Model file for the job. Use its own axes, mm. A direction names the side the tool comes from. Give positions to 0.01 mm unless a question says otherwise; leave off trailing zeros. Write each loop counter-clockwise with the first axis right and the second up, starting at its lowest first coordinate (ties: lowest second). Pieces come first, ordered by that corner, then holes. Notation, with made-up numbers: (72.25, -10) - (128.25, -10) arc R32 ccw to (128.25, 23) - close; hole circle Ø4 at (3, 42.5). An arc over 180 degrees is marked (long way). One line per item, written item: value. Start each with the question number.
(1) Mould opens along X. For faces 6 (the face through (-47.622, 0.74, 30.417)), 7 (the face through (65.665, 5.979, 35.509)), 8 (the face through (5, 2, 39.516)) say: pulls with the +X half, pulls with the -X half, needs draft (parallel to the pull), parting line crosses it, or undercut.
(2) Cut at A-A, the plane y = 6.25. List the corners of the cut face in (x, z), and give its area (3 significant figures).
(3) Cut at D-D, the plane z = 5. List the corners of the cut face in (x, y), and give its area (3 significant figures).
(4) Cut at C-C, the plane z = -14. List the corners of the cut face in (x, y), and give its area (3 significant figures).
(5) Drop flat-ended pins along their axis: P1, Ø5, axis at x = 60, z = -54.5, coming from the +Y side; P2, Ø1.8, axis at x = -49, z = -56, coming from the -Y side; P3, Ø0.9, axis at x = -16.5, y = 6.5, coming from the +Z side; P4, Ø1.8, axis at x = 59.52, z = 29.52, coming from the -Y side. Give the stop position or say it passes through.
(6) Cut at B-B, the plane x = 39.5. List the corners of the cut face in (y, z), and give its area (3 significant figures).
(7) Probe L1, parallel to X at y = 6.25, z = -35; L2, parallel to Z at x = 6, y = 6; L3, parallel to X at y = 0.5, z = 32. List the from-to ranges inside material, lowest first.
(8) 3-axis set-ups, long thin cutter, end or side, ignore diameter. For faces 1 (the face through (-56.63, 5.98, -61.48)), 2 (the face through (4, 6, -64.484)), 3 (the face through (34, 2, -21.699)), 4 (the face through (62.378, 0.74, 30.417)), 5 (the face through (64.665, 5.979, 34.509)): which of +Z, -Z, +X, -X, +Y, -Y reach the whole face in a straight line?
from build123d import *

# Parameters (mm, degrees)
SKETCH_1_R          = 6.5
EXTRUDE_1_DEPTH     = 4.5
EXTRUDE_2_DEPTH     = 3
SKETCH_3_R          = 1
CUT_EXTRUDE_1_DEPTH = 10
SKETCH_4_R          = 3
CUT_EXTRUDE_2_DEPTH = 1
SKETCH_5_R          = 3
CUT_EXTRUDE_3_DEPTH = 1.5
SKETCH_6_W          = 19.238645782
SKETCH_6_H          = 11.749776954
CUT_EXTRUDE_6_DEPTH = 10


with BuildPart() as part:
    # 草图1 → 凸台-拉伸1 (new body)
    with BuildSketch(Plane(origin=(0, 0, 0), x_dir=(1, 0, 0), z_dir=(0, 1, 0))):
        with BuildLine():
            Line((-50.483870968, 65.483870968), (59.516129032, 65.483870968))
            ThreePointArc((59.516129032, 65.483870968), (66.587196844, 62.55493878), (69.516129032, 55.483870968))
            Line((69.516129032, 55.483870968), (69.516129032, -29.516129032))
            ThreePointArc((69.516129032, -29.516129032), (66.587196844, -36.587196844), (59.516129032, -39.516129032))
            Line((59.516129032, -39.516129032), (-50.483870968, -39.516129032))
            ThreePointArc((-50.483870968, -39.516129032), (-57.55493878, -36.587196844), (-60.483870968, -29.516129032))
            Line((-60.483870968, -29.516129032), (-60.483870968, 55.483870968))
            ThreePointArc((-60.483870968, 55.483870968), (-57.55493878, 62.55493878), (-50.483870968, 65.483870968))
        make_face()
        with Locations((-0.483870968, 15.483870968)):
            Circle(SKETCH_1_R, mode=Mode.SUBTRACT)
    extrude(amount=EXTRUDE_1_DEPTH)

    # 草图2 → 凸台-拉伸2 (add)
    with BuildSketch(Plane(origin=(0, 4.5, 0), x_dir=(1, 0, 0), z_dir=(0, 1, 0))):
        with BuildLine():
            Line((-49.483870968, 64.483870968), (58.516129032, 64.483870968))
            ThreePointArc((58.516129032, 64.483870968), (65.587196844, 61.55493878), (68.516129032, 54.483870968))
            Line((68.516129032, 54.483870968), (68.516129032, -28.516129032))
            ThreePointArc((68.516129032, -28.516129032), (65.587196844, -35.587196844), (58.516129032, -38.516129032))
            Line((58.516129032, -38.516129032), (-49.483870968, -38.516129032))
            ThreePointArc((-49.483870968, -38.516129032), (-56.55493878, -35.587196844), (-59.483870968, -28.516129032))
            Line((-59.483870968, -28.516129032), (-59.483870968, 54.483870968))
            ThreePointArc((-59.483870968, 54.483870968), (-56.55493878, 61.55493878), (-49.483870968, 64.483870968))
        make_face()
        with BuildLine():
            Line((-48.483870968, 63.483870968), (57.516129032, 63.483870968))
            ThreePointArc((57.516129032, 63.483870968), (64.587196844, 60.55493878), (67.516129032, 53.483870968))
            Line((67.516129032, 53.483870968), (67.516129032, -27.516129032))
            ThreePointArc((67.516129032, -27.516129032), (64.587196844, -34.587196844), (57.516129032, -37.516129032))
            Line((57.516129032, -37.516129032), (-48.483870968, -37.516129032))
            ThreePointArc((-48.483870968, -37.516129032), (-55.55493878, -34.587196844), (-58.483870968, -27.516129032))
            Line((-58.483870968, -27.516129032), (-58.483870968, 53.483870968))
            ThreePointArc((-58.483870968, 53.483870968), (-55.55493878, 60.55493878), (-48.483870968, 63.483870968))
        make_face(mode=Mode.SUBTRACT)
    extrude(amount=EXTRUDE_2_DEPTH)

    # 草图3 → 切除-拉伸1 (cut)
    with BuildSketch(Plane(origin=(0, 4.5, 0), x_dir=(1, 0, 0), z_dir=(0, 1, 0))):
        with Locations((-50.483870968, 55.483870968)):
            Circle(SKETCH_3_R)
        with Locations((-50.483870968, -29.516129032)):
            Circle(SKETCH_3_R)
        with Locations((59.516129032, -29.516129032)):
            Circle(SKETCH_3_R)
        with Locations((59.516129032, 55.483870968)):
            Circle(SKETCH_3_R)
    extrude(amount=-CUT_EXTRUDE_1_DEPTH, mode=Mode.SUBTRACT)

    # 草图4 → 切除-拉伸2 (cut)
    with BuildSketch(Plane(origin=(0, 4.5, 0), x_dir=(1, 0, 0), z_dir=(0, 1, 0))):
        with Locations((-50.483870968, 55.483870968)):
            Circle(SKETCH_4_R)
        with Locations((59.516129032, 55.483870968)):
            Circle(SKETCH_4_R)
        with Locations((59.516129032, -29.516129032)):
            Circle(SKETCH_4_R)
        with Locations((-50.483870968, -29.516129032)):
            Circle(SKETCH_4_R)
    extrude(amount=-CUT_EXTRUDE_2_DEPTH, mode=Mode.SUBTRACT)

    # 草图5 → 切除-拉伸3 (cut)
    with BuildSketch(Plane.XZ):
        with Locations((-50.483870968, 29.516129032)):
            Circle(SKETCH_5_R)
        with Locations((59.516129032, 29.516129032)):
            Circle(SKETCH_5_R)
        with Locations((59.516129032, -55.483870968)):
            Circle(SKETCH_5_R)
        with Locations((-50.483870968, -55.483870968)):
            Circle(SKETCH_5_R)
    extrude(amount=-CUT_EXTRUDE_3_DEPTH, mode=Mode.SUBTRACT)

    # 草图6 → 切除-拉伸6 (cut)
    with BuildSketch(Plane(origin=(0, 4.5, 0), x_dir=(1, 0, 0), z_dir=(0, 1, 0))):
        with Locations((34.019689846, 15.824476385)):
            Rectangle(SKETCH_6_W, SKETCH_6_H)
    extrude(amount=-CUT_EXTRUDE_6_DEPTH, mode=Mode.SUBTRACT)


solid = part.part
Answers follow:
1. face 6: undercut
1. face 7: pulls with the +X half
1. face 8: needs draft
2. outline: (-59.48, -54.48) arc R10 ccw to (-49.48, -64.48) - (58.52, -64.48) arc R10 ccw to (68.52, -54.48) - (68.52, 28.52) arc R10 ccw to (58.52, 38.52) - (-49.48, 38.52) arc R10 ccw to (-59.48, 28.52) - close; hole (-58.48, -53.48) arc R10 ccw to (-48.48, -63.48) - (57.52, -63.48) arc R10 ccw to (67.52, -53.48) - (67.52, 27.52) arc R10 ccw to (57.52, 37.52) - (-48.48, 37.52) arc R10 ccw to (-58.48, 27.52) - close
2. area: 458 mm²
3. outline: (-60.48, 0) - (69.52, 0) - (69.52, 4.5) - (68.52, 4.5) - (68.52, 7.5) - (67.52, 7.5) - (67.52, 4.5) - (-58.48, 4.5) - (-58.48, 7.5) - (-59.48, 7.5) - (-59.48, 4.5) - (-60.48, 4.5) - close
3. area: 591 mm²
4. outline: (-60.48, 0) - (-6.81, 0) - (-6.81, 4.5) - (-58.48, 4.5) - (-58.48, 7.5) - (-59.48, 7.5) - (-59.48, 4.5) - (-60.48, 4.5) - close; (5.84, 0) - (24.4, 0) - (24.4, 4.5) - (5.84, 4.5) - close; (43.64, 0) - (69.52, 0) - (69.52, 4.5) - (68.52, 4.5) - (68.52, 7.5) - (67.52, 7.5) - (67.52, 4.5) - (43.64, 4.5) - close
4. area: 447 mm²
5. P1: stops at y = 4.5
5. P2: stops at y = 1.5
5. P3: stops at z = 38.52
5. P4: passes through
6. outline: (0, -65.48) - (4.5, -65.48) - (4.5, -64.48) - (7.5, -64.48) - (7.5, -63.48) - (4.5, -63.48) - (4.5, -21.7) - (0, -21.7) - close; (0, -9.95) - (4.5, -9.95) - (4.5, 37.52) - (7.5, 37.52) - (7.5, 38.52) - (4.5, 38.52) - (4.5, 39.52) - (0, 39.52) - close
6. area: 426 mm²
7. L1: x = -59.48 to -58.48, 67.52 to 68.52
7. L2: z = -64.48 to -63.48, 37.52 to 38.52
7. L3: x = -60.17 to -52.17, -48.8 to 57.83, 61.2 to 69.2
8. face 1: -Z, -X, +Y
8. face 2: -Z, +X, -X, +Y
8. face 3: +Y, -Y
8. face 4: -Y
8. face 5: +Y
